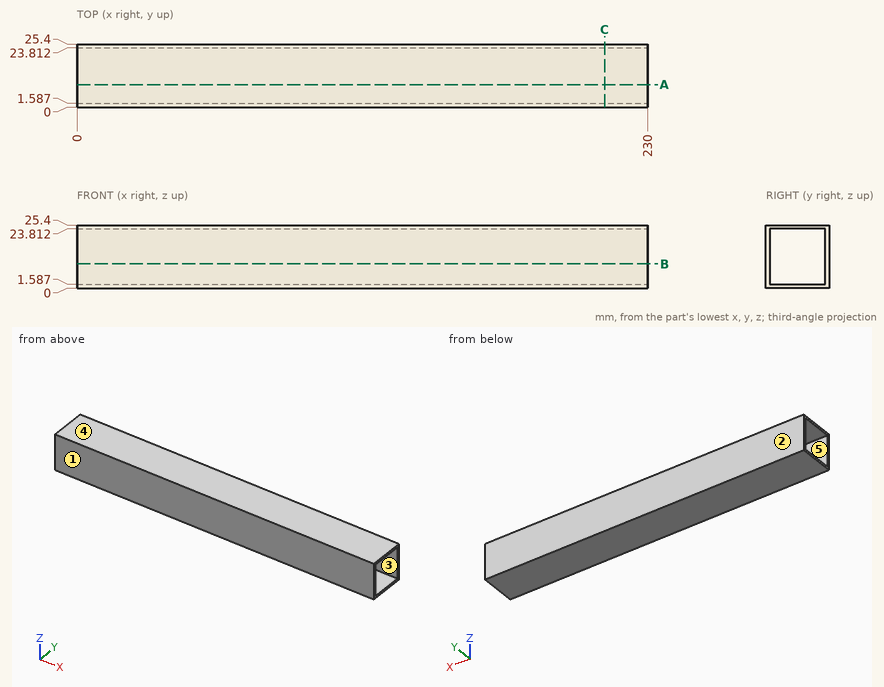
Answer from the drawing. Dimensions are ordinates in mm from the lowest x, y and z of the part. A direction names the side the tool comes from. Give positions to 0.01 mm unless a question says otherwise; leave off trailing zeros. Write each loop counter-clockwise with the first axis right and the second up, starting at its lowest first coordinate (ties: lowest second). Pieces come first, ordered by that corner, then holes. Notation, with made-up numbers: M 73.5,-12 L 84.5,-12 A28 cw 84.5,18 Z; hole C -32,22 d1. An arc over 180 degrees is marked long. Answer as CSV lines item,"result".
Q1. A tool of negligible diameter and unlimited length cuts with its end or side. For the marked faces 4 and 5, from which of +Z, -Z, +X, -X, +Y, -Y can it reach the whole face along a straight path? Write none if from no direction.
A:
face 4,"+Z, +X, -X, +Y, -Y"
face 5,"+X, -X"
Q2. A cutting plane is placed at C-C on x = 212.5. Write down the section's boundary in (y, z).
A:
outline,"M 0,0 L 25.4,0 L 25.4,25.4 L 0,25.4 Z; hole M 1.59,1.59 L 23.81,1.59 L 23.81,23.81 L 1.59,23.81 Z"
Q3. The mould has two halves that part along Y. Classify the marked faces 1, 2 and 3: +Y half, -Y half, draft (parallel to the pull), parting line (faces both ways), or undercut.
A:
face 1,"-Y half"
face 2,"+Y half"
face 3,"undercut"
Q4. A cutting plane is placed at A-A on y = 9. Write down the section's boundary in (x, z).
A:
outline,"M 0,0 L 230,0 L 230,1.59 L 0,1.59 Z; M 0,23.81 L 230,23.81 L 230,25.4 L 0,25.4 Z"
Q5. Find the intervals of material crossed by probe 1 along Z at (x, y) = (21, 18), in increasing order. Write a range as [from, to].
A:
probe 1,"z = [0, 1.59], [23.81, 25.4]"
